Can you work these out from the model? Positions are in its coordinate system, mm. Coordinates: 2 decimals unless noted, no trailing zeros. Order: outer loops, then holes, each group sorted by start corner. A loop starts at its lowest first (then second) coordinate and runs counter-clockwise, first axis right, second up. Notation, with made-up numbers: (-4, 82) -> (45, 82) arc R25 cw to (45, 104) -> close; hole circle Ø2 at (75.25, 32.5). An arc over 180 degrees is marked (long way). Use a Markdown table: item, result. Add a question column.
1. If I drill on line 1 along Z through (x, y) = (2.4, 71.5); line 2 along Z through (x, y) = (1.5, -4); line 3 along Y through (x, z) = (2.1, 12), over which ranges is the centre line in solid material (lowest first)? Write a range as from..to.
2. Suppose I cut it at A-A, the plane z = 32.5. List the corners of the cut face in (x, y) for me.
3. Suppose I cut it at B-B, the plane x = 1.5. List the corners of the cut face in (y, z) for me.
4. Suppose I cut it at D-D, the plane y = 318. List the corners of the cut face in (x, z) for me.
5. Suppose I cut it at C-C, the plane y = -78.5. List the corners of the cut face in (x, z) for me, then the cut area to 3 significant figures.
6. We'd pull the mould along Y, two halves only. Please class faces 1 (the flat face through (1.252, 91.73, 158.426)), 2 (the flat face through (1.25, 129.69, 196.24)), 3 (the flat face through (0, 63, 58)): pulls with the +Y half, pulls with the -Y half, needs draft (parallel to the pull), parting line crosses it, or undercut.
7. For pin 1 Ø1.3 at (x, y) = (1.5, 153.5) entering from +Z; pin 2 Ø1.5 at (x, z) = (0.5, 234.5) entering from +Y, each with a flat end and sliding along its axis, tell me the tip position at first contact or that it passes through.
```python
from build123d import *

# Parameters (mm, degrees)
SKETCH1_W           = 127
SKETCH1_H           = 431.8
BOSS_EXTRUDE1_DEPTH = 2.54


with BuildPart() as part:
    # Sketch1 → Boss-Extrude1 (new body)
    with BuildSketch(Plane(origin=(0, 0, 0), x_dir=(0, 0, -1), z_dir=(1, 0, 0))):
        Polygon((-67.465907198, 387.242597926), (135.734092802, 387.242597926), (135.734092802, -146.157402074), (-321.465907198, -146.157402074), (-321.465907198, -120.757402074), align=None)
        with Locations((21.434092802, 120.542597926)):
            Rectangle(SKETCH1_W, SKETCH1_H, mode=Mode.SUBTRACT)
        Polygon((-67.465907198, 273.650344669), (-251.969780569, -95.357402074), (-67.465907198, -95.357402074), align=None, mode=Mode.SUBTRACT)
    extrude(amount=BOSS_EXTRUDE1_DEPTH)


solid = part.part
```
Worked out:
| question | item | result |
|---|---|---|
| 1 | line 1 | z = -135.73..-84.93, 42.07..67.47, 168.54..225.34 |
| 1 | line 2 | z = -135.73..-84.93, 42.07..67.47, 206.29..263.09 |
| 1 | line 3 | y = -146.16..-95.36, 336.44..387.24 |
| 2 | outline | (0, -146.16) -> (2.54, -146.16) -> (2.54, -95.36) -> (0, -95.36) -> close; (0, 336.44) -> (2.54, 336.44) -> (2.54, 387.24) -> (0, 387.24) -> close |
| 3 | outline | (-146.16, -135.73) -> (387.24, -135.73) -> (387.24, 67.47) -> (-120.76, 321.47) -> (-146.16, 321.47) -> close; hole (-95.36, -84.93) -> (336.44, -84.93) -> (336.44, 42.07) -> (-95.36, 42.07) -> close; hole (-95.36, 67.47) -> (273.65, 67.47) -> (-95.36, 251.97) -> close |
| 4 | outline | (0, -135.73) -> (2.54, -135.73) -> (2.54, -84.93) -> (0, -84.93) -> close; (0, 42.07) -> (2.54, 42.07) -> (2.54, 102.09) -> (0, 102.09) -> close |
| 5 | outline | (0, -135.73) -> (2.54, -135.73) -> (2.54, -84.93) -> (0, -84.93) -> close; (0, 42.07) -> (2.54, 42.07) -> (2.54, 67.47) -> (0, 67.47) -> close; (0, 243.54) -> (2.54, 243.54) -> (2.54, 300.34) -> (0, 300.34) -> close |
| 5 | area | 338 mm² |
| 6 | face 1 | undercut |
| 6 | face 2 | pulls with the +Y half |
| 6 | face 3 | needs draft |
| 7 | pin 1 | stops at z = 184.66 |
| 7 | pin 2 | stops at y = 54.67 |
